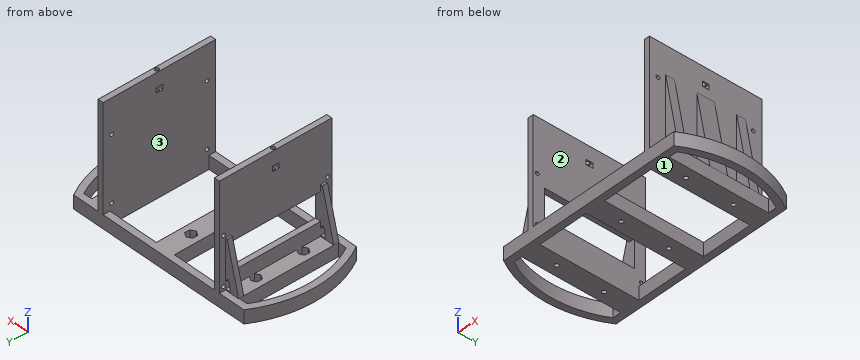
```python
from build123d import *

# Parameters (mm, degrees)
SKETCH1_W                = 152.4
SKETCH1_H                = 101.6
BOSS_EXTRUDE1_DEPTH      = 12
F_6_CLEARANCE_HOLE1_D    = 3.7973
BOSS_EXTRUDE2_DEPTH      = 12
CUT_EXTRUDE2_DEPTH       = 9.525
SKETCH5_W                = 46.008
SKETCH5_H                = 89.6
CUT_EXTRUDE1_DEPTH       = 112.353602017
SKETCH7_W                = 5
SKETCH7_H                = 101.6
BOSS_EXTRUDE3_DEPTH      = 50.8
M3_CLEARANCE_HOLE1_D     = 3.4
SKETCH9_W                = 25.4
SKETCH9_H                = 81.28
CUT_EXTRUDE3_DEPTH       = 174.339792114
BOSS_EXTRUDE4_START      = -45.29
BOSS_EXTRUDE4_DEPTH      = 4.65
BOSS_EXTRUDE4_START_2    = 40.64
BOSS_EXTRUDE4_2_DEPTH    = 4.65
CUT_EXTRUDE4_DEPTH       = 152.169152879
SKETCH12_W               = 5
SKETCH12_H               = 101.6
BOSS_EXTRUDE5_DEPTH      = 70
M3_CLEARANCE_HOLE2_D     = 3.4
M3_CLEARANCE_HOLE2_DEPTH = 43.3535
BOSS_EXTRUDE6_REACH      = 193.164
SKETCH14_W               = 71.196910045
SKETCH14_H               = 16
SKETCH14_H_2             = 8
BOSS_EXTRUDE7_DEPTH      = 25
BOSS_EXTRUDE8_REACH      = 155.963
SKETCH16_W               = 5
SKETCH16_H               = 101.6
SKETCH17_R               = 1.75
CUT_EXTRUDE5_DEPTH       = 20
CUT_EXTRUDE6_DEPTH       = 198.763845357
CUT_EXTRUDE6_DEPTH_BACK  = 198.763845357
SKETCH19_W               = 4.5
SKETCH19_H               = 6


# Read off the part's stored shape, not the designer's step: Boss-Extrude4
with BuildPart() as part:
    # Sketch1 → Boss-Extrude1 (new body)
    with BuildSketch(Plane.XY):
        Rectangle(SKETCH1_W, SKETCH1_H)
    extrude(amount=BOSS_EXTRUDE1_DEPTH)

    # #6 Clearance Hole1 (through all)
    with Locations(Plane(origin=(-64.008, 21.46427, 12), x_dir=(1, 0, 0), z_dir=(0, 0, 1))):
        with Locations((0, 0), (128.016, 0), (128.016, -42.92854), (0, -42.92854), (64.008, 0), (64.008, -42.92854)):
            Hole(F_6_CLEARANCE_HOLE1_D / 2)

    # Sketch4 → Boss-Extrude2 (add)
    with BuildSketch(Plane.XY.offset(12)):
        with BuildLine():
            Line((-76.2, 50.8), (-84.22793291, 50.8))
            ThreePointArc((-84.22793291, 50.8), (-98.3615, 0), (-84.22793291, -50.8))
            Line((-84.22793291, -50.8), (-76.2, -50.8))
            Line((-76.2, -50.8), (-76.2, 50.8))
        make_face()
        with BuildLine():
            Line((76.2, -50.8), (84.22793291, -50.8))
            ThreePointArc((84.22793291, -50.8), (98.3615, 0), (84.22793291, 50.8))
            Line((84.22793291, 50.8), (76.2, 50.8))
            Line((76.2, 50.8), (76.2, -50.8))
        make_face()
    extrude(amount=-BOSS_EXTRUDE2_DEPTH)

    # Sketch6 → Cut-Extrude2 (cut)
    with BuildSketch(Plane.XY.offset(12)):
        Polygon((-68.008, 19.154868923), (-64.008, 16.845467846), (-60.008, 19.154868923), (-60.008, 23.773671077), (-64.008, 26.083072154), (-68.008, 23.773671077), align=None)
        Polygon((4, 19.154868923), (4, 23.773671077), (0, 26.083072154), (-4, 23.773671077), (-4, 19.154868923), (0, 16.845467846), align=None)
        Polygon((68.008, 19.154868923), (68.008, 23.773671077), (64.008, 26.083072154), (60.008, 23.773671077), (60.008, 19.154868923), (64.008, 16.845467846), align=None)
        Polygon((68.008, -23.773671077), (68.008, -19.154868923), (64.008, -16.845467846), (60.008, -19.154868923), (60.008, -23.773671077), (64.008, -26.083072154), align=None)
        Polygon((4, -23.773671077), (4, -19.154868923), (0, -16.845467846), (-4, -19.154868923), (-4, -23.773671077), (0, -26.083072154), align=None)
        Polygon((-60.008, -23.773671077), (-60.008, -19.154868923), (-64.008, -16.845467846), (-68.008, -19.154868923), (-68.008, -23.773671077), (-64.008, -26.083072154), align=None)
    extrude(amount=-CUT_EXTRUDE2_DEPTH, mode=Mode.SUBTRACT)

    # Sketch5 → Cut-Extrude1 (cut, through all)
    with BuildSketch(Plane.XY.offset(12)):
        with BuildLine():
            Line((-73.008, 44.8), (-73.008, -44.8))
            Line((-73.008, -44.8), (-80.768847226, -44.8))
            ThreePointArc((-80.768847226, -44.8), (-92.3615, 0), (-80.768847226, 44.8))
            Line((-80.768847226, 44.8), (-73.008, 44.8))
        make_face()
        with BuildLine():
            Line((73.008, 44.8), (73.008, -44.8))
            Line((73.008, -44.8), (80.768847226, -44.8))
            ThreePointArc((80.768847226, -44.8), (92.3615, 0), (80.768847226, 44.8))
            Line((80.768847226, 44.8), (73.008, 44.8))
        make_face()
        with Locations((-32.004, 0)):
            Rectangle(SKETCH5_W, SKETCH5_H)
        with Locations((32.004, 0)):
            Rectangle(SKETCH5_W, SKETCH5_H)
    extrude(amount=-CUT_EXTRUDE1_DEPTH, mode=Mode.SUBTRACT)

    # Sketch7 → Boss-Extrude3 (add)
    with BuildSketch(Plane.XY.offset(12)):
        with Locations((-57.508, 0)):
            Rectangle(SKETCH7_W, SKETCH7_H)
    extrude(amount=BOSS_EXTRUDE3_DEPTH)

    # M3 Clearance Hole1 (through all)
    with Locations(Plane(origin=(-55.008, 46.99, 58.99), x_dir=(0, 1, 0), z_dir=(1, 0, 0))):
        with Locations((0, 0), (0, -43.18), (-93.98, -43.18), (-93.98, 0)):
            Hole(M3_CLEARANCE_HOLE1_D / 2)

    # Sketch9 → Cut-Extrude3 (cut, through all)
    with BuildSketch(Plane(origin=(-55.008, 0, 0), x_dir=(0, 0, -1), z_dir=(1, 0, 0))):
        with Locations((-37.4, 0)):
            Rectangle(SKETCH9_W, SKETCH9_H)
    extrude(amount=-CUT_EXTRUDE3_DEPTH, mode=Mode.SUBTRACT)

    # Boss-Extrude4 outline → Boss-Extrude4 (add)
    with BuildSketch(Plane(origin=(0, 0, 0), x_dir=(1, 0, 0), z_dir=(0, 1, 0)).offset(BOSS_EXTRUDE4_START)):
        Polygon((-60.008, -12), (-73.008, -12), (-60.008, -62.8), align=None)
    extrude(amount=BOSS_EXTRUDE4_DEPTH)

    # Boss-Extrude4 2 outline → Boss-Extrude4 2 (add)
    with BuildSketch(Plane(origin=(0, 0, 0), x_dir=(1, 0, 0), z_dir=(0, 1, 0)).offset(BOSS_EXTRUDE4_START_2)):
        Polygon((-60.008, -12), (-73.008, -12), (-60.008, -62.8), align=None)
    extrude(amount=BOSS_EXTRUDE4_2_DEPTH)

    # Sketch11 → Cut-Extrude4 (cut, through all)
    with BuildSketch(Plane(origin=(0, -45.29, 0), x_dir=(-1, 0, 0), z_dir=(0, -1, 0))):
        Polygon((64.508, -18.81), (62.258, -22.707114317), (60.008, -18.81), (60.008, -12.81), (64.508, -12.81), align=None)
        Polygon((60.008, -55.99), (64.508, -55.99), (64.508, -61.99), (64.508, -62.8), (60.008, -62.8), (60.008, -61.99), align=None)
    extrude(amount=-CUT_EXTRUDE4_DEPTH, mode=Mode.SUBTRACT)

    # Sketch12 → Boss-Extrude5 (add)
    with BuildSketch(Plane.XY.offset(12)):
        with Locations((57.508, 0)):
            Rectangle(SKETCH12_W, SKETCH12_H)
    extrude(amount=BOSS_EXTRUDE5_DEPTH)

    # M3 Clearance Hole2
    with Locations(Plane(origin=(55.008, -43, 76), x_dir=(0, -1, 0), z_dir=(-1, 0, 0))):
        with Locations((0, 0), (0, -58), (-86, -58), (-86, 0)):
            Hole(M3_CLEARANCE_HOLE2_D / 2, depth=M3_CLEARANCE_HOLE2_DEPTH)

    # Boss-Extrude6: up to this face of the body (flat: up to its plane)
    boss_extrude6_end = Plane(part.part.faces().sort_by_distance((60.008, 0, 46.511614943))[0])
    # Sketch14 → Boss-Extrude6 (add, up to the picked face)
    with BuildSketch(Plane(origin=(72.728190965, 0, 13.506664036), x_dir=(-0.18259219384277645, 0, 0.983188736076488), z_dir=(-0.9831887360764879, 0, -0.18259219384277642)), mode=Mode.PRIVATE) as boss_extrude6_sk1:
        with Locations((34.066028968, 0)):
            Rectangle(SKETCH14_W, SKETCH14_H)
    boss_extrude6_tool1 = split(extrude(boss_extrude6_sk1.sketch, amount=BOSS_EXTRUDE6_REACH, mode=Mode.PRIVATE), bisect_by=boss_extrude6_end, keep=Keep.BOTH, mode=Mode.PRIVATE)
    # Sketch14 → Boss-Extrude6 (add, up to the picked face)
    with BuildSketch(Plane(origin=(72.728190965, 0, 13.506664036), x_dir=(-0.18259219384277645, 0, 0.983188736076488), z_dir=(-0.9831887360764879, 0, -0.18259219384277642)), mode=Mode.PRIVATE) as boss_extrude6_sk2:
        with Locations((34.066028968, -32.083072154)):
            Rectangle(SKETCH14_W, SKETCH14_H_2)
    boss_extrude6_tool2 = split(extrude(boss_extrude6_sk2.sketch, amount=BOSS_EXTRUDE6_REACH, mode=Mode.PRIVATE), bisect_by=boss_extrude6_end, keep=Keep.BOTH, mode=Mode.PRIVATE)
    # Sketch14 → Boss-Extrude6 (add, up to the picked face)
    with BuildSketch(Plane(origin=(72.728190965, 0, 13.506664036), x_dir=(-0.18259219384277645, 0, 0.983188736076488), z_dir=(-0.9831887360764879, 0, -0.18259219384277642)), mode=Mode.PRIVATE) as boss_extrude6_sk3:
        with Locations((34.066028968, 32.083072154)):
            Rectangle(SKETCH14_W, SKETCH14_H_2)
    boss_extrude6_tool3 = split(extrude(boss_extrude6_sk3.sketch, amount=BOSS_EXTRUDE6_REACH, mode=Mode.PRIVATE), bisect_by=boss_extrude6_end, keep=Keep.BOTH, mode=Mode.PRIVATE)
    add(boss_extrude6_tool1.solids().sort_by(Axis((66.508, 0, 47), (-0.9831887360764879, 0, -0.18259219384277642)))[0])
    add(boss_extrude6_tool2.solids().sort_by(Axis((66.508, -32.083072, 47), (-0.9831887360764879, 0, -0.18259219384277642)))[0])
    add(boss_extrude6_tool3.solids().sort_by(Axis((66.508, 32.083072, 47), (-0.9831887360764879, 0, -0.18259219384277642)))[0])

    # Sketch15 → Boss-Extrude7 (add)
    with BuildSketch(Plane.XY.offset(82)):
        Polygon((60.008, 50.8), (55.008, 50.8), (55.008, -50.8), (60.008, -50.8), (60.008, -36.083072154), (60.008, -28.083072154), (60.008, -8), (60.008, 8), (60.008, 28.083072154), (60.008, 36.083072154), align=None)
    extrude(amount=BOSS_EXTRUDE7_DEPTH)

    # Sketch16 → Boss-Extrude8 (add, up to next)
    with BuildSketch(Plane.XY.offset(107), mode=Mode.PRIVATE) as boss_extrude8_sk1:
        with Locations((-57.508, 0)):
            Rectangle(SKETCH16_W, SKETCH16_H)
    boss_extrude8_tool1 = extrude(boss_extrude8_sk1.sketch, amount=-BOSS_EXTRUDE8_REACH, mode=Mode.PRIVATE) - part.part
    add(boss_extrude8_tool1.solids().sort_by_distance((-57.508, 0, 107))[0])

    # Sketch17 → Cut-Extrude5 (cut)
    with BuildSketch(Plane.XY.offset(107)):
        with Locations((-57.508, 0)):
            Circle(SKETCH17_R)
        with Locations((57.508, 0)):
            Circle(SKETCH17_R)
    extrude(amount=-CUT_EXTRUDE5_DEPTH, mode=Mode.SUBTRACT)

    # Sketch19 → Cut-Extrude6 (cut, two sides: drawn at the far end of the back side and taken through both)
    with BuildSketch(Plane.ZY.offset(60.008).offset(-CUT_EXTRUDE6_DEPTH_BACK)):
        with Locations((92, 0)):
            Rectangle(SKETCH19_W, SKETCH19_H)
    extrude(amount=CUT_EXTRUDE6_DEPTH + CUT_EXTRUDE6_DEPTH_BACK, mode=Mode.SUBTRACT)


solid = part.part
```
Work out the finished part from the listing and answer in its coordinate system (mm). Face numbers are marked on the shaded views. Give positions to 0.01 mm unless a question says otherwise; leave off trailing zeros. Order: outer loops, then holes, each group sorted by start corner. A loop starts at its lowest first (then second) coordinate and runs counter-clockwise, first axis right, second up. Notation, with made-up numbers: (68, 15) -> (116, 15) arc R23 cw to (116, 30) -> close; hole circle Ø9 at (11.25, 13). An arc over 180 degrees is marked (long way). Answer as CSV lines item,"result". Start each with the question number.
(1) Section D-D, the plane z = 36.5 is taken. Write down the section's boundary in (x, y), plus the area to 3 significant figures.
(2) For a pull along X with two mould halves and no side action, classify the marked faces 1, 2 and 3 as released by +X, released by -X, zero draft, split by the parting line, or undercut.
(3) Section A-A, the plane x = -40.5 is taken. Write down the section's boundary in (y, z), plus the area to 3 significant figures.
(4) Section B-B, the plane z = 66 is taken. Write down the section's boundary in (x, y).
(5) Section C-C, the plane y = 12 is taken. Write down the section's boundary in (x, z).
(6) Each of these flat-tipped pins is pushed along its axis until it touches: pin 1 Ø6.5 at (x, y) = (69.5, 20) entering from +Z; pin 2 Ø1.9 at (x, y) = (-61.5, -43.5) entering from +Z; pin 3 Ø6 at (y, z) = (-6.5, 7) entering from -X; pin 4 Ø12 at (x, y) = (17.5, 4) entering from +Z. Where does it stop, or does it pass through?
(7) Consider line 1 along Y through (x, z) = (0, 1); line 2 along Y through (x, z) = (62, 54); line 3 along X through (y, z) = (-23.5, 24). Determine where each line is inside the solid, lowest interval first.
Entries:
1,outline,"(-66.74, -45.29) -> (-60.01, -45.29) -> (-60.01, -50.8) -> (-55.01, -50.8) -> (-55.01, -40.64) -> (-66.74, -40.64) -> close; (-66.74, 40.64) -> (-55.01, 40.64) -> (-55.01, 50.8) -> (-60.01, 50.8) -> (-60.01, 45.29) -> (-66.74, 45.29) -> close; (55.01, -50.8) -> (60.01, -50.8) -> (60.01, -36.08) -> (68.46, -36.08) -> (68.46, -28.08) -> (60.01, -28.08) -> (60.01, -8) -> (68.46, -8) -> (68.46, 8) -> (60.01, 8) -> (60.01, 28.08) -> (68.46, 28.08) -> (68.46, 36.08) -> (60.01, 36.08) -> (60.01, 50.8) -> (55.01, 50.8) -> close"
1,area,"943 mm²"
2,face 1,"zero draft"
2,face 2,"undercut"
2,face 3,"undercut"
3,outline,"(-50.8, 0) -> (-44.8, 0) -> (-44.8, 12) -> (-50.8, 12) -> close; (44.8, 0) -> (50.8, 0) -> (50.8, 12) -> (44.8, 12) -> close"
3,area,"144 mm²"
4,outline,"(-60.01, -50.8) -> (-55.01, -50.8) -> (-55.01, 50.8) -> (-60.01, 50.8) -> close; (55.01, -50.8) -> (60.01, -50.8) -> (60.01, -36.08) -> (62.98, -36.08) -> (62.98, -28.08) -> (60.01, -28.08) -> (60.01, -8) -> (62.98, -8) -> (62.98, 8) -> (60.01, 8) -> (60.01, 28.08) -> (62.98, 28.08) -> (62.98, 36.08) -> (60.01, 36.08) -> (60.01, 50.8) -> (55.01, 50.8) -> close"
5,outline,"(-97.63, 0) -> (-91.58, 0) -> (-91.58, 12) -> (-97.63, 12) -> close; (-73.01, 0) -> (-55.01, 0) -> (-55.01, 24.7) -> (-60.01, 24.7) -> (-60.01, 12) -> (-73.01, 12) -> close; (-60.01, 50.1) -> (-55.01, 50.1) -> (-55.01, 107) -> (-60.01, 107) -> close; (-9, 0) -> (9, 0) -> (9, 12) -> (-9, 12) -> close; (55.01, 0) -> (73.01, 0) -> (73.01, 12) -> (60.01, 12) -> (60.01, 107) -> (55.01, 107) -> close; (91.58, 0) -> (97.63, 0) -> (97.63, 12) -> (91.58, 12) -> close"
6,pin 1,"z = 12"
6,pin 2,"z = 55.99"
6,pin 3,"x = -98.3"
6,pin 4,"through"
7,line 1,"-50.8 to -23.36, -19.57 to 19.57, 23.36 to 50.8"
7,line 2,"-36.08 to -28.08, -8 to 8, 28.08 to 36.08"
7,line 3,"-60.01 to -55.01, 55.01 to 60.01"
